The listing builds one solid part. Answer for the finished solid, in the listing's coordinates (mm). A direction names the side the tool comes from. Give positions to 0.01 mm unless a question says otherwise; leave off trailing zeros. Write each loop counter-clockwise with the first axis right and the second up, starting at its lowest first coordinate (ties: lowest second). Pieces come first, ordered by that corner, then holes. Notation, with made-up numbers: M 4,88.5 L 34,88.5 A18 ccw 34,93.5 Z; hole C 84,19 d2. An arc over 180 degrees is marked long. Answer as a JSON object with one key per item and string values.
```python
from build123d import *

# Parameters (mm, degrees)
BOSS_EXTRUDE1_DEPTH     = 1.498487888
SKETCH2_R               = 1.5
CUT_EXTRUDE1_DEPTH      = 2.498487888
CUT_EXTRUDE2_DEPTH      = 2.498487888
LPATTERN1_COUNT         = 2
LPATTERN1_PITCH         = 9.525
MIRROR1_COPY_1_SKETCH_R = 1.5
MIRROR1_COPY_1_DEPTH    = 2.498487888


with BuildPart() as part:
    # Sketch1 → Boss-Extrude1 (new body)
    with BuildSketch(Plane(origin=(0, 0, 0), x_dir=(1, 0, 0), z_dir=(0, 1, 0))):
        Polygon((-57.15, -11.1125), (-38.1, -17.4625), (38.1, -17.4625), (57.15, -11.1125), (57.15, 17.4625), (19.05, 17.4625), (15.875, 4.7625), (-15.875, 4.7625), (-19.05, 17.4625), (-57.15, 17.4625), align=None)
    extrude(amount=BOSS_EXTRUDE1_DEPTH)

    # Sketch2 → Cut-Extrude1 (cut, through all)
    with BuildSketch(Plane(origin=(0, 1.498487888, 0), x_dir=(1, 0, 0), z_dir=(0, 1, 0))):
        with Locations((-53.975, 14.2875)):
            Circle(SKETCH2_R)
        with Locations((-28.575, 14.2875)):
            Circle(SKETCH2_R)
    cut_extrude1 = extrude(amount=-CUT_EXTRUDE1_DEPTH, mode=Mode.SUBTRACT)

    # Sketch5 → Cut-Extrude2 (cut, through all)
    with BuildSketch(Plane(origin=(0, 1.498487888, 0), x_dir=(1, 0, 0), z_dir=(0, 1, 0))):
        Polygon((-50.8, 17.4625), (-47.625, 11.1125), (-34.925, 11.1125), (-31.75, 17.4625), align=None)
    cut_extrude2 = extrude(amount=-CUT_EXTRUDE2_DEPTH, mode=Mode.SUBTRACT)

    # LPattern1: Cut-Extrude1 ×2
    with Locations(*[(0, 0, i * LPATTERN1_PITCH) for i in range(1, LPATTERN1_COUNT)]):
        add(cut_extrude1, mode=Mode.SUBTRACT)

    # Mirror1: Cut-Extrude2, Cut-Extrude1 across plane
    add(cut_extrude2.mirror(Plane(origin=(0, 0, 0), x_dir=(0, 0, 1), z_dir=(1, 0, 0))), mode=Mode.SUBTRACT)
    add(cut_extrude1.mirror(Plane(origin=(0, 0, 0), x_dir=(0, 0, 1), z_dir=(1, 0, 0))), mode=Mode.SUBTRACT)

    # Mirror1 copy 1 sketch → Mirror1 copy 1 (cut, through all)
    with BuildSketch(Plane(origin=(0, 1.498487888, 9.525), x_dir=(-1, 0, 0), z_dir=(0, 1, 0))):
        with Locations((-53.975, -14.2875)):
            Circle(MIRROR1_COPY_1_SKETCH_R)
        with Locations((-28.575, -14.2875)):
            Circle(MIRROR1_COPY_1_SKETCH_R)
    extrude(amount=-MIRROR1_COPY_1_DEPTH, mode=Mode.SUBTRACT)


solid = part.part
```
1. A flat-ended cylindrical pin translates along its axis: pin 1 (0.7 mm diameter, centred on x = -39, y = 1, fed in from -Z). Find the tip coordinate at first contact, or state that the pin passes through.
Verdict:
{"pin 1": "stops at z = -11.11"}
2. A cutting plane is placed at B-B, the plane y = 1. Count the separate pieces of the cut face and the enclosed holes in it, plus the area to 3 significant figures.
Verdict:
{"separate pieces": "1", "enclosed holes": "8", "area": "3,170 mm2"}
3. A cutting plane is placed at C-C, the plane x = -14. Give the vertices of the cut face in (y, z), plus the area to 3 significant figures.
Verdict:
{"outline": "M 0,-4.76 L 1.5,-4.76 L 1.5,17.46 L 0,17.46 Z", "area": "33.3 mm2"}
4. A cutting plane is placed at A-A, the plane z = -8. Give the vertices of the cut face in (x, y), plus the area to 3 significant figures.
Verdict:
{"outline": "M -57.15,0 L -16.68,0 L -16.68,1.5 L -57.15,1.5 Z; M 16.68,0 L 57.15,0 L 57.15,1.5 L 16.68,1.5 Z", "area": "121 mm2"}
5. For faces 4 (the cylindrical face through (27.144, 0.76, -4.312)), 5 (the flat face through (49.235, 0.76, -14.332)), determine the directions among +Z, -Z, +X, -X, +Y, -Y from which every point of the face is accessible in a straight line to the end or side of a thin tool.
Verdict:
{"face 4": "+Y, -Y", "face 5": "-Z, +Y, -Y"}
6. A cutting plane is placed at D-D, the plane x = 17. Give the vertices of the cut face in (y, z), plus the area to 3 significant figures.
Verdict:
{"outline": "M 0,-9.26 L 1.5,-9.26 L 1.5,17.46 L 0,17.46 Z", "area": "40.0 mm2"}
7. The mould has two halves that part along Z. Classify faces 1 (the flat face through (47.492, 0.739, 14.332)), 2 (the cylindrical face through (-53.169, 0.76, -15.552)), 3 (the flat face through (-1, 1.498, 4)): released by +Z, released by -Z, zero draft, split by the parting line, or undercut.
Verdict:
{"face 1": "released by +Z", "face 2": "undercut", "face 3": "zero draft"}
8. Consider line 1 along X through (y, z) = (0.7, -5.5); line 2 along Z through (x, y) = (-3.5, 0.15); line 3 along X through (y, z) = (1.1, -3.5) (3 decimals). Determine where each line is inside the solid, lowest interval first.
Verdict:
{"line 1": "x = -57.15 to -55.28, -52.67 to -29.88, -27.27 to -16.06, 16.06 to 27.27, 29.88 to 52.67, 55.28 to 57.15", "line 2": "z = -4.76 to 17.46", "line 3": "x = -57.15 to -54.785, -53.165 to -29.385, -27.765 to 27.765, 29.385 to 53.165, 54.785 to 57.15"}
